Could you check a few things on this drawing? It's one solid part, dimensions in mm from its lowest x, y, z. Round coordinates to 2 decimals unless told otherwise and drop trailing zeros. Order: outer loops, then holes, each group sorted by start corner. A loop starts at its lowest first (then second) coordinate and runs counter-clockwise, first axis right, second up. Notation, with made-up numbers: M -9,23 L 50,23 A10 ccw 50,37 Z; hole C 78.5,19 d9. An arc over 180 degrees is marked long. Answer as a JSON object with one key per item and string values. Group by question number.
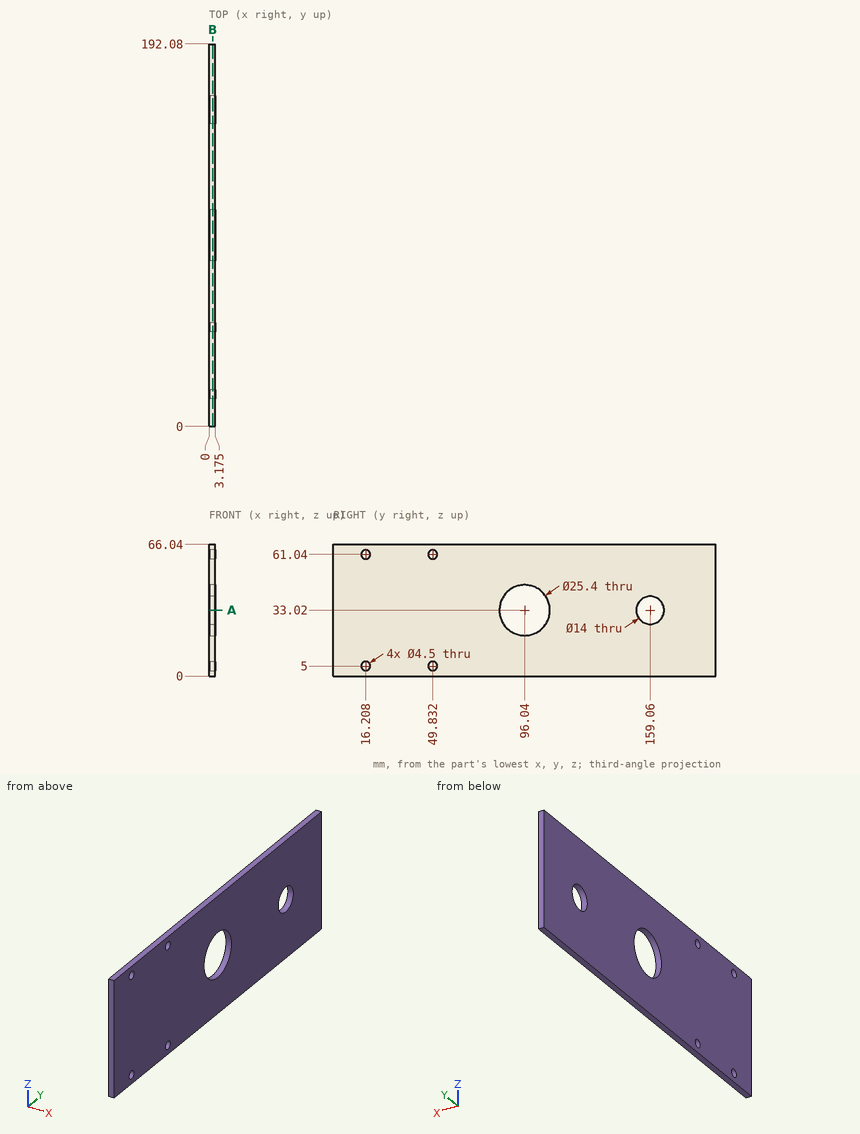
1) I need wall thicknesses on line 1 along Y through (x, z) = (1, 33.02); line 2 along Y through (x, z) = (2.1, 6); line 3 along Z through (x, y) = (2.5, 14.5) (1 decimal). Which ranges of each line are inside material? Lowest first, please.
2) If we section it at B-B on x = 1.75: Write out the boundary of the cut face in (y, z), plus the area to 3 significant figures.
3) If we section it at A-A on z = 33.02: Write out the boundary of the cut face in (x, y) (3 decimals), plus the area to 3 significant figures.
Findings:
{
 "1": {"line 1": "y = 0 to 83.34, 108.74 to 152.06, 166.06 to 192.08", "line 2": "y = 0 to 14.19, 18.22 to 47.82, 51.85 to 192.08", "line 3": "z = 0 to 3.5, 6.5 to 59.6, 62.5 to 66"},
 "2": {"outline": "M 0,0 L 192.08,0 L 192.08,66.04 L 0,66.04 Z; hole C 16.21,5 d4.5; hole C 16.21,61.04 d4.5; hole C 49.83,5 d4.5; hole C 49.83,61.04 d4.5; hole C 96.04,33.02 d25.4; hole C 159.06,33.02 d14", "area": "12,000 mm^2"},
 "3": {"outline": "M 0,0 L 3.175,0 L 3.175,83.34 L 0,83.34 Z; M 0,108.74 L 3.175,108.74 L 3.175,152.06 L 0,152.06 Z; M 0,166.06 L 3.175,166.06 L 3.175,192.08 L 0,192.08 Z", "area": "485 mm^2"}
}
